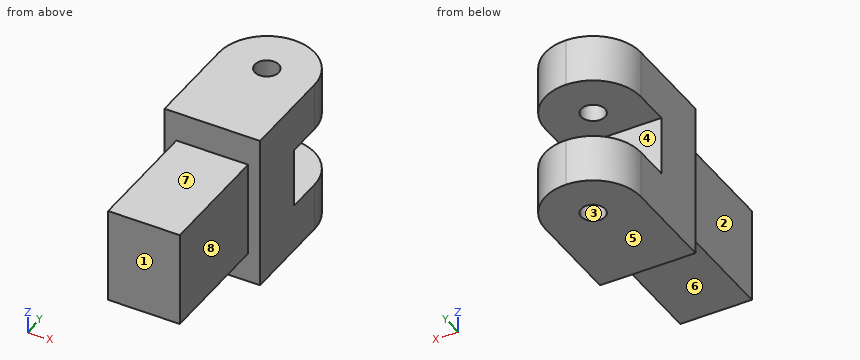
from build123d import *

# Parameters (mm, degrees)
SKETCH1_W           = 8
SKETCH1_H           = 13
BOSS_EXTRUDE1_DEPTH = 12
SKETCH2_W           = 13
SKETCH2_H           = 5
CUT_EXTRUDE1_DEPTH  = 7
SKETCH3_R           = 1
CUT_EXTRUDE2_DEPTH  = 19.138357147
CUT_EXTRUDE3_START  = -13
CUT_EXTRUDE3_DEPTH  = 32.138357147
SKETCH6_W           = 6
SKETCH6_H           = 8
BOSS_EXTRUDE3_DEPTH = 10


with BuildPart() as part:
    # Sketch1 → Boss-Extrude1 (new body)
    with BuildSketch(Plane(origin=(0, 0, 0), x_dir=(1, 0, 0), z_dir=(0, 1, 0))):
        Rectangle(SKETCH1_W, SKETCH1_H)
    extrude(amount=BOSS_EXTRUDE1_DEPTH)

    # Sketch2 → Cut-Extrude1 (cut)
    with BuildSketch(Plane(origin=(0, 12, 0), x_dir=(1, 0, 0), z_dir=(0, 1, 0))):
        Rectangle(SKETCH2_W, SKETCH2_H)
    extrude(amount=-CUT_EXTRUDE1_DEPTH, mode=Mode.SUBTRACT)

    # Sketch3 → Cut-Extrude2 (cut, through all)
    with BuildSketch(Plane(origin=(0, 0, -6.5), x_dir=(-1, 0, 0), z_dir=(0, 0, -1))):
        with Locations((0, 8)):
            Circle(SKETCH3_R)
    extrude(amount=-CUT_EXTRUDE2_DEPTH, mode=Mode.SUBTRACT)

    # Sketch4 → Cut-Extrude3 (cut)
    with BuildSketch(Plane(origin=(0, 0, -6.5), x_dir=(-1, 0, 0), z_dir=(0, 0, -1)).offset(CUT_EXTRUDE3_START)):
        with BuildLine():
            Line((-4, -27.298221281), (-4, 8))
            ThreePointArc((-4, 8), (-2.828427125, 10.828427125), (0, 12))
            Line((0, 12), (35.298221281, 12))
            Line((35.298221281, 12), (-14.621001982, 61.919223264))
            Line((-14.621001982, 61.919223264), (-53.919223264, 22.621001982))
            Line((-53.919223264, 22.621001982), (-4, -27.298221281))
        make_face()
    cut_extrude3 = extrude(amount=CUT_EXTRUDE3_DEPTH, mode=Mode.SUBTRACT)

    # Mirror1: Cut-Extrude3 across plane
    add(cut_extrude3.mirror(Plane(origin=(0, 0, 0), x_dir=(0, 0, 1), z_dir=(1, 0, 0))), mode=Mode.SUBTRACT)

    # Sketch6 → Boss-Extrude3 (add)
    with BuildSketch(Plane.XZ):
        Rectangle(SKETCH6_W, SKETCH6_H)
    extrude(amount=BOSS_EXTRUDE3_DEPTH)


solid = part.part
Geometry check sheet. Reference: the model listing, model coordinates, mm. Face numbers are marked on the shaded views. A direction names the side the tool comes from. Round coordinates to 2 decimals unless told otherwise and drop trailing zeros. Loops run counter-clockwise (first coordinate to the right, second up) from the corner with the lowest first, then second, coordinate; pieces in that order, holes last. Notation, with made-up numbers: (-17, 40.25) -> (3, 40.25) arc R22 ccw to (3, 58.25) -> close; hole circle Ø1 at (3, 18). An arc over 180 degrees is marked (long way). Answer as a JSON object with one key per item and string values. Group by question number.
Item 1: Cross-section at B-B, the plane y = 7.5. Record the cut outline in (x, z).
Item 2: Cross-section at D-D, the plane y = 9.75. Record the cut outline in (x, z), plus the area to 4 significant figures.
Item 3: Release check for a two-part mould opening along X. For the marked faces 1, 2 and 3 record: pulls with the +X half, pulls with the -X half, needs draft (parallel to the pull), parting line crosses it, or undercut.
Item 4: Cross-section at A-A, the plane z = 3.25. Record the cut outline in (x, y), plus the area to 3 significant figures.
Item 5: Thickness scan on line 1 along Z through (x, y) = (0.5, 6.75); line 2 along Y through (x, z) = (0, 4.25); line 3 along X through (y, z) = (-9, -0.5). Record the ranges inside material, lowest first.
Item 6: Cross-section at C-C, the plane z = -2.25. Record the cut outline in (x, y), plus the area to 3 significant figures.
Item 7: Set-up check for the marked faces 4, 5, 6, 7 and 8: record each of +Z, -Z, +X, -X, +Y, -Y from which the full face is reachable in a straight line by a thin tool's end or side.
Item 8: Depth check by flat-ended pin: pin 1 Ø3 at (x, y) = (-1, -3) entering from -Z; pin 2 Ø4 at (y, z) = (-5, -0.5) entering from +X. Enter the tip coordinate at first touch or a pass-through.
Determined:
{
 "1": {"outline": "(-4, -6.5) -> (-0.87, -6.5) -> (-0.87, -2.5) -> (-4, -2.5) -> close; (-4, 2.5) -> (-0.87, 2.5) -> (-0.87, 6.5) -> (-4, 6.5) -> close; (0.87, -6.5) -> (4, -6.5) -> (4, -2.5) -> (0.87, -2.5) -> close; (0.87, 2.5) -> (4, 2.5) -> (4, 6.5) -> (0.87, 6.5) -> close"},
 "2": {"outline": "(-3.6, -6.5) -> (3.6, -6.5) -> (3.6, -2.5) -> (-3.6, -2.5) -> close; (-3.6, 2.5) -> (3.6, 2.5) -> (3.6, 6.5) -> (-3.6, 6.5) -> close", "area": "57.55 mm²"},
 "3": {"face 1": "needs draft", "face 2": "pulls with the -X half", "face 3": "undercut"},
 "4": {"outline": "(-4, 0) -> (-3, 0) -> (-3, -10) -> (3, -10) -> (3, 0) -> (4, 0) -> (4, 8) arc R4 ccw to (-4, 8) -> close; hole circle Ø2 at (0, 8)", "area": "146 mm²"},
 "5": {"line 1": "z = -6.5 to -2.5, 2.5 to 6.5", "line 2": "y = 0 to 7, 9 to 12", "line 3": "x = -3 to 3"},
 "6": {"outline": "(-4, 0) -> (-3, 0) -> (-3, -10) -> (3, -10) -> (3, 0) -> (4, 0) -> (4, 5) -> (-4, 5) -> close", "area": "100 mm²"},
 "7": {"face 4": "+X, -X, +Y", "face 5": "-Z, +X, -X, +Y, -Y", "face 6": "-Z, +X, -X, -Y", "face 7": "+Z, +X, -X, -Y", "face 8": "+Z, -Z, +X, -Y"},
 "8": {"pin 1": "stops at z = -4", "pin 2": "stops at x = 3"}
}
